from build123d import *

# Parameters (mm, degrees)
SKETCH_1_W             = 87
SKETCH_1_H             = 15
EXTRUDE_1_DEPTH        = 22
SKETCH_2_W             = 8
SKETCH_2_H             = 15
CUT_EXTRUDE_1_DEPTH    = 8
SKETCH_3_W             = 8
SKETCH_3_H             = 12.5
CUT_EXTRUDE_2_DEPTH    = 1
SKETCH_4_W             = 1.5
SKETCH_4_H             = 6.8
CUT_EXTRUDE_3_DEPTH    = 1
FILLET_1_R             = 1
SKETCH_5_W             = 7.25
SKETCH_5_H             = 12
EXTRUDE_2_DEPTH        = 2
FILLET_2_R             = 2
PATTERN_LINEAR_1_COUNT = 9
PATTERN_LINEAR_1_PITCH = 9.5
FILLET_3_R             = 1
FILLET_4_R             = 2
CUT_EXTRUDE_4_DEPTH    = 36


with BuildPart() as part:
    # Эскиз1 → Бобышка-Вытянуть1 (new body)
    with BuildSketch(Plane.XY):
        Rectangle(SKETCH_1_W, SKETCH_1_H)
    extrude(amount=EXTRUDE_1_DEPTH)

    # Эскиз2 → Вырез-Вытянуть1 (cut)
    with BuildSketch(Plane(origin=(0, 0, 0), x_dir=(-1, 0, 0), z_dir=(0, 0, -1))):
        with Locations((-38, 0)):
            Rectangle(SKETCH_2_W, SKETCH_2_H)
        with Locations((-28.5, 0)):
            Rectangle(SKETCH_2_W, SKETCH_2_H)
        with Locations((-19, 0)):
            Rectangle(SKETCH_2_W, SKETCH_2_H)
        with Locations((-9.5, 0)):
            Rectangle(SKETCH_2_W, SKETCH_2_H)
        Rectangle(SKETCH_2_W, SKETCH_2_H)
        with Locations((9.5, 0)):
            Rectangle(SKETCH_2_W, SKETCH_2_H)
        with Locations((19, 0)):
            Rectangle(SKETCH_2_W, SKETCH_2_H)
        with Locations((28.5, 0)):
            Rectangle(SKETCH_2_W, SKETCH_2_H)
        with Locations((38, 0)):
            Rectangle(SKETCH_2_W, SKETCH_2_H)
    extrude(amount=-CUT_EXTRUDE_1_DEPTH, mode=Mode.SUBTRACT)

    # Эскиз3 → Вырез-Вытянуть2 (cut)
    with BuildSketch(Plane.XZ.offset(7.5)):
        with Locations((-38, 14.25)):
            Rectangle(SKETCH_3_W, SKETCH_3_H)
        with Locations((-28.5, 14.25)):
            Rectangle(SKETCH_3_W, SKETCH_3_H)
        with Locations((-19, 14.25)):
            Rectangle(SKETCH_3_W, SKETCH_3_H)
        with Locations((-9.5, 14.25)):
            Rectangle(SKETCH_3_W, SKETCH_3_H)
        with Locations((0, 14.25)):
            Rectangle(SKETCH_3_W, SKETCH_3_H)
        with Locations((9.5, 14.25)):
            Rectangle(SKETCH_3_W, SKETCH_3_H)
        with Locations((19, 14.25)):
            Rectangle(SKETCH_3_W, SKETCH_3_H)
        with Locations((28.5, 14.25)):
            Rectangle(SKETCH_3_W, SKETCH_3_H)
        with Locations((38, 14.25)):
            Rectangle(SKETCH_3_W, SKETCH_3_H)
    extrude(amount=-CUT_EXTRUDE_2_DEPTH, mode=Mode.SUBTRACT)

    # Эскиз4 → Вырез-Вытянуть3 (cut)
    with BuildSketch(Plane.XZ.offset(7.5)):
        with Locations((-33.25, 3.4)):
            Rectangle(SKETCH_4_W, SKETCH_4_H)
        with Locations((-23.75, 3.4)):
            Rectangle(SKETCH_4_W, SKETCH_4_H)
        with Locations((-14.25, 3.4)):
            Rectangle(SKETCH_4_W, SKETCH_4_H)
        with Locations((-4.75, 3.4)):
            Rectangle(SKETCH_4_W, SKETCH_4_H)
        with Locations((4.75, 3.4)):
            Rectangle(SKETCH_4_W, SKETCH_4_H)
        with Locations((14.25, 3.4)):
            Rectangle(SKETCH_4_W, SKETCH_4_H)
        with Locations((23.75, 3.4)):
            Rectangle(SKETCH_4_W, SKETCH_4_H)
        with Locations((33.25, 3.4)):
            Rectangle(SKETCH_4_W, SKETCH_4_H)
        with Locations((42.75, 3.4)):
            Rectangle(SKETCH_4_W, SKETCH_4_H)
    extrude(amount=-CUT_EXTRUDE_3_DEPTH, mode=Mode.SUBTRACT)

    # Скругление1
    fillet_1_edges = [part.edges().sort_by_distance(p)[0] for p in [
        (42.75, -7.5, 6.8),
        (33.25, -7.5, 6.8),
        (23.75, -7.5, 6.8),
        (14.25, -7.5, 6.8),
        (4.75, -7.5, 6.8),
        (-4.75, -7.5, 6.8),
        (-14.25, -7.5, 6.8),
        (-23.75, -7.5, 6.8),
        (-33.25, -7.5, 6.8),
    ]]
    fillet(fillet_1_edges, radius=FILLET_1_R - 0.0001)  # a hair under: the kernel refuses the full size

    # Эскиз5 → Бобышка-Вытянуть2 (add)
    with BuildSketch(Plane(origin=(0, 0, 8), x_dir=(-1, 0, 0), z_dir=(0, 0, -1))):
        with Locations((-28.5, 0.5)):
            Rectangle(SKETCH_5_W, SKETCH_5_H)
        with Locations((-38, 0.5)):
            Rectangle(SKETCH_5_W, SKETCH_5_H)
        with Locations((-19, 0.5)):
            Rectangle(SKETCH_5_W, SKETCH_5_H)
        with Locations((-9.5, 0.5)):
            Rectangle(SKETCH_5_W, SKETCH_5_H)
        with Locations((0, 0.5)):
            Rectangle(SKETCH_5_W, SKETCH_5_H)
        with Locations((9.5, 0.5)):
            Rectangle(SKETCH_5_W, SKETCH_5_H)
        with Locations((19, 0.5)):
            Rectangle(SKETCH_5_W, SKETCH_5_H)
        with Locations((28.5, 0.5)):
            Rectangle(SKETCH_5_W, SKETCH_5_H)
        with Locations((38, 0.5)):
            Rectangle(SKETCH_5_W, SKETCH_5_H)
    extrude(amount=EXTRUDE_2_DEPTH)

    # Скругление2
    fillet_2_edges = [part.edges().sort_by_distance(p)[0] for p in [
        (38, 6.5, 6),
        (38, -5.5, 6),
        (28.5, 6.5, 6),
        (28.5, -5.5, 6),
        (19, 6.5, 6),
        (9.5, -5.5, 6),
        (19, -5.5, 6),
        (9.5, 6.5, 6),
        (0, 6.5, 6),
        (0, -5.5, 6),
        (-9.5, 6.5, 6),
        (-9.5, -5.5, 6),
        (-19, 6.5, 6),
        (-19, -5.5, 6),
        (-28.5, 6.5, 6),
        (-38, 6.5, 6),
        (-28.5, -5.5, 6),
        (-38, -5.5, 6),
    ]]
    fillet(fillet_2_edges, radius=FILLET_2_R - 0.0001)  # a hair under: the kernel refuses the full size

    # Эскиз6 → Отверстие обработанное метчиком M31 (revolve, cut)
    with BuildSketch(Plane(origin=(-38, 0, 6), x_dir=(0, 1, 0), z_dir=(1, 0, 0))):
        Polygon((0, 0), (0, 6.251075774), (1.25, 5.5), (1.25, 0), align=None)
    hole_wizard_m31 = revolve(axis=Axis((-38, 0, -0.35), (0, 0, 1)), mode=Mode.SUBTRACT)

    # Линейный массив1: Отверстие обработанное метчиком M31 ×9
    with Locations(*[(i * PATTERN_LINEAR_1_PITCH, 0, 0) for i in range(1, PATTERN_LINEAR_1_COUNT)]):
        add(hole_wizard_m31, mode=Mode.SUBTRACT)

    # Скругление3
    fillet_3_edges = [part.edges().sort_by_distance(p)[0] for p in [
        (42.75, -6.5, 0),
        (-42.75, -7.5, 0),
    ]]
    fillet(fillet_3_edges, radius=FILLET_3_R)

    # Скругление4
    fillet_4_edges = [part.edges().sort_by_distance(p)[0] for p in [
        (-33.25, -6.5, 0),
        (-23.75, -6.5, 0),
        (-14.25, -6.5, 0),
        (-4.75, -6.5, 0),
        (4.75, -6.5, 0),
        (14.25, -6.5, 0),
        (23.75, -6.5, 0),
        (33.25, -6.5, 0),
    ]]
    fillet(fillet_4_edges, radius=FILLET_4_R)

    # Эскиз8 → Вырез-Вытянуть4 (cut, symmetric)
    with BuildSketch(Plane(origin=(0, 0, 0), x_dir=(0, 0, -1), z_dir=(1, 0, 0))):
        with BuildLine():
            Line((-1.8, 7.5), (0.321320344, 7.5))
            Line((0.321320344, 7.5), (0.321320344, 7.2))
            ThreePointArc((0.321320344, 7.2), (-0.739339828, 6.760660172), (-1.8, 7.2))
            Line((-1.8, 7.2), (-1.8, 7.5))
        make_face()
    extrude(amount=CUT_EXTRUDE_4_DEPTH, both=True, mode=Mode.SUBTRACT)


solid = part.part
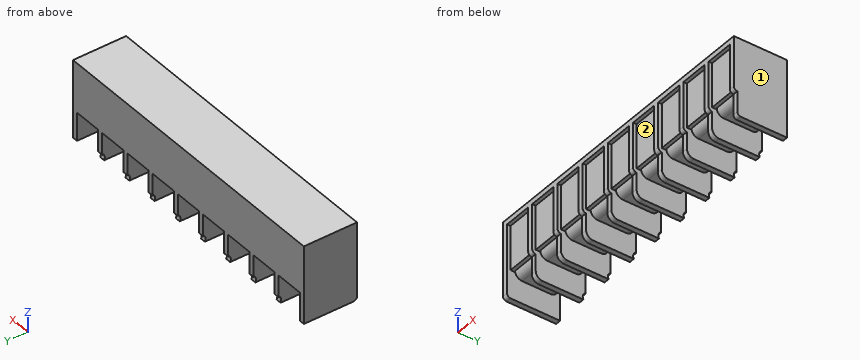
Input: part model. Units: mm. Frame: model coordinates. Face numbers are marked on the shaded views. A direction names the side the tool comes from. Coordinates: 2 decimals unless noted, no trailing zeros. Answer as CSV lines item,"result".
1. First-contact query: P1, Ø3, axis at x = 9.5, y = 0, coming from the -Z side; P2, Ø2, axis at x = -9.5, y = 0, coming from the -Z side; P3, Ø5, axis at x = -29, z = 17.5, coming from the -Y side. Flat tips, straight axial feed; report the tip coordinate or a pass-through.
Reported:
P1,"z = 6"
P2,"z = 11.65"
P3,"y = -6.5"
2. Material intervals for line 1 (Y direction, x = -38, z = 8.5); line 2 (Z direction, x = 6, y = 0); line 3 (Z direction, x = -36.5, y = -7), sorted ascending. Write a range as from..to.
Reported:
line 1,"-6.5..-1.25, 1.25..7.5"
line 2,"6..22"
line 3,"20.5..22"
3. Access query for the marked faces 1 and 2. Directions: +Z, -Z, +X, -X, +Y, -Y. A direction counts if a zero-diameter tool reaches every point of the face in a straight line with its end or side. Return the directions, or none.
Reported:
face 1,"+Z, -Z, +X, +Y, -Y"
face 2,"-Z, -Y"
